Geometry check sheet. Reference: the model listing, model coordinates, mm. A direction names the side the tool comes from. Coordinates: 2 decimals unless noted, no trailing zeros. Order: outer loops, then holes, each group sorted by start corner. A loop starts at its lowest first (then second) coordinate and runs counter-clockwise, first axis right, second up. Notation, with made-up numbers: (8.5, 77) - (56.5, 77) arc R25 cw to (56.5, 102) - close; hole circle Ø7 at (-33.75, 38). An arc over 180 degrees is marked (long way). Return JSON: item names as keys, results as strings. Group by question number.
Item 1: Section check D-D on x = -18. Enter the section's corners in (y, z) (3 decimals), then the cut area to 3 significant figures.
Item 2: Gauge pin test, flat ends, axial feed: pin 1 (2.5 mm diameter, centred on y = 15.5, z = -6.5, fed in from +X); pin 2 (1.7 mm diameter, centred on x = 2.5, y = 4, fed in from +Z); pin 3 (8 mm diameter, centred on y = 20.5, z = 6, fed in from -X); pin 4 (12 mm diameter, centred on x = 6.5, z = -6.5, fed in from -Y). Record the tip position at first contact, or that the pin passes through.
Item 3: Section check B-B on y = 6.75. Enter the section's corners in (x, z) (3 decimals).
Item 4: Draft check along X on faces 6 (the cylindrical face through (-21.555, 5.114, -19.879)), 7 (the flat face through (23, 1, -20.5)), 8 (the cylindrical face through (26.886, 1.166, -0.208)), 9 (the flat face through (28.3, 1, 0)). Enter one of: pulls with the +X half, pulls with the -X half, needs draft (parallel to the pull), parting line crosses it, or undercut.
Item 5: Scan lines: probe 1 along Y at (x, z) = (-24.5, -6.5); probe 2 along X at (y, z) = (1.4, -17.5); probe 3 along Z at (x, y) = (-15, 6). Record each from-to range of solid material in increasing order.
Item 6: Section check C-C on z = -17.5. Enter the section's corners in (x, y) (3 decimals), then the cut area to 3 significant figures.
Item 7: Tool access check on faces 1 (the cylindrical face through (23.237, 5.114, 3.452)), 2 (the flat face through (-21.693, 12.255, 3.512)), 3 (the flat face through (23, 1, 20.5)), 4 (the flat face through (-25, 5, -13.02)), 5 (the flat face through (-22.125, 5, 17)). Record the directions out of +Z, -Z, +X, -X, +Y, -Y that give a thin tool (end or side, any length) a straight path to the whole face; none if there is none.
Item 8: Section check A-A on x = -25.3. Enter the section's corners in (y, z) (3 decimals).
from build123d import *

# Parameters (mm, degrees)
SKETCH1_W               = 56.6
SKETCH1_H               = 41
BOSS_EXTRUDE1_DEPTH     = 2.3
BOSS_EXTRUDE2_DEPTH     = 5.55
BOSS_EXTRUDE3_DEPTH     = 15.15
FILLET1_R               = 2
BOSS_EXTRUDE5_DEPTH     = 2.3
BOSS_EXTRUDE6_DEPTH     = 2.3
SKETCH6_R               = 1.6
CUT_EXTRUDE1_DEPTH      = 42.199956917
FILLET2_R               = 3.5
SKETCH7_R               = 4.708157521
BOSS_EXTRUDE7_DEPTH     = 0.2
SKETCH11_R              = 4.425
BOSS_EXTRUDE8_DEPTH     = 2.45
CUT_EXTRUDE2_DEPTH      = 10
CUT_EXTRUDE2_DEPTH_BACK = 2.45
SKETCH12_R              = 3.925
BOSS_EXTRUDE10_DEPTH    = 1


with BuildPart() as part:
    # Sketch1 → Boss-Extrude1 (new body)
    with BuildSketch(Plane(origin=(0, 0, 0), x_dir=(1, 0, 0), z_dir=(0, 1, 0))):
        Rectangle(SKETCH1_W, SKETCH1_H)
    extrude(amount=BOSS_EXTRUDE1_DEPTH)

    # Sketch2 → Boss-Extrude2 (add)
    with BuildSketch(Plane(origin=(0, 2.3, 0), x_dir=(1, 0, 0), z_dir=(0, 1, 0))):
        Polygon((-22.125, -20.48), (28.285, -20.48), (28.285, -4.45), (22.185, -4.45), (22.185, 4.45), (28.285, 4.45), (28.285, 20.48), (-22.125, 20.48), (-22.125, 13.02), (-28.285, 13.02), (-28.285, -13.02), (-22.125, -13.02), align=None)
    extrude(amount=BOSS_EXTRUDE2_DEPTH)

    # Sketch3 → Boss-Extrude3 (add)
    with BuildSketch(Plane(origin=(0, 7.85, 0), x_dir=(1, 0, 0), z_dir=(0, 1, 0))):
        with BuildLine():
            Line((-19, -18.225), (21, -18.225))
            ThreePointArc((21, -18.225), (22.185, 0), (21, 18.225))
            Line((21, 18.225), (-19, 18.225))
            ThreePointArc((-19, 18.225), (-20.414213562, 17.639213562), (-21, 16.225))
            Line((-21, 16.225), (-21, -16.225))
            ThreePointArc((-21, -16.225), (-20.414213562, -17.639213562), (-19, -18.225))
        make_face()
    extrude(amount=BOSS_EXTRUDE3_DEPTH)

    # Fillet1
    fillet1_edges = [part.edges().sort_by_distance(p)[0] for p in [
        (28.285, 5.075, -20.48),
        (-22.125, 5.075, -20.48),
        (-22.125, 5.075, -13.02),
        (-28.285, 5.075, -13.02),
        (-28.285, 5.075, 13.02),
        (-22.125, 5.075, 13.02),
        (-22.125, 5.075, 20.48),
        (28.285, 5.075, 20.48),
        (28.3, 1.15, 20.5),
        (-28.3, 1.15, 20.5),
        (-28.3, 1.15, -20.5),
        (28.3, 1.15, -20.5),
    ]]
    fillet(fillet1_edges, radius=FILLET1_R)

    # Sketch4 → Boss-Extrude5 (add)
    with BuildSketch(Plane(origin=(0, 0, 0), x_dir=(1, 0, 0), z_dir=(0, 1, 0))):
        with BuildLine():
            Line((28.3, 14.772353725), (28.3, 9.587646275))
            ThreePointArc((28.3, 9.587646275), (28.429084519, 10.095465182), (28.785, 10.48))
            Line((28.785, 10.48), (28.785, 13.88))
            ThreePointArc((28.785, 13.88), (28.429084519, 14.264534818), (28.3, 14.772353725))
        make_face()
        with BuildLine():
            ThreePointArc((28.3, -9.587646275), (28.429084519, -10.095465182), (28.785, -10.48))
            Line((28.785, -10.48), (28.785, -13.88))
            ThreePointArc((28.785, -13.88), (28.429084519, -14.264534818), (28.3, -14.772353725))
            Line((28.3, -14.772353725), (28.3, -9.587646275))
        make_face()
    extrude(amount=BOSS_EXTRUDE5_DEPTH)

    # Sketch5 → Boss-Extrude6 (add)
    with BuildSketch(Plane(origin=(29.434734965, 0, -17.005006325), x_dir=(0, 0, -1), z_dir=(0, 1, 0))):
        with BuildLine():
            Line((3.494993675, 9.629302498), (3.494993675, 9.486266265))
            ThreePointArc((3.494993675, 9.486266265), (3.620682756, 10.143155137), (3.979993675, 10.707244136))
            Line((3.979993675, 10.707244136), (3.979993675, 14.149734965))
            ThreePointArc((3.979993675, 14.149734965), (3.621827878, 14.636664087), (3.494993675, 15.227676603))
            Line((3.494993675, 15.227676603), (3.494993675, 9.629302498))
        make_face()
        with BuildLine():
            Line((-37.505006325, 46.813203664), (-37.505006325, 46.670167432))
            Line((-37.505006325, 46.670167432), (-37.505006325, 41.071793326))
            ThreePointArc((-37.505006325, 41.071793326), (-37.631840527, 41.662805842), (-37.990006325, 42.149734965))
            Line((-37.990006325, 42.149734965), (-37.990006325, 45.592225793))
            ThreePointArc((-37.990006325, 45.592225793), (-37.630695406, 46.156314792), (-37.505006325, 46.813203664))
        make_face()
        with BuildLine():
            Line((3.494993675, 41.071793326), (3.494993675, 46.670167432))
            Line((3.494993675, 46.670167432), (3.494993675, 46.813203664))
            ThreePointArc((3.494993675, 46.813203664), (3.620682756, 46.156314792), (3.979993675, 45.592225793))
            Line((3.979993675, 45.592225793), (3.979993675, 42.149734965))
            ThreePointArc((3.979993675, 42.149734965), (3.621827878, 41.662805842), (3.494993675, 41.071793326))
        make_face()
        with BuildLine():
            Line((-37.505006325, 15.227676603), (-37.505006325, 9.629302498))
            Line((-37.505006325, 9.629302498), (-37.505006325, 9.486266265))
            ThreePointArc((-37.505006325, 9.486266265), (-37.630695406, 10.143155137), (-37.990006325, 10.707244136))
            Line((-37.990006325, 10.707244136), (-37.990006325, 14.149734965))
            ThreePointArc((-37.990006325, 14.149734965), (-37.631840527, 14.636664087), (-37.505006325, 15.227676603))
        make_face()
    extrude(amount=BOSS_EXTRUDE6_DEPTH)

    # Sketch6 → Cut-Extrude1 (cut, through all)
    with BuildSketch(Plane(origin=(0, 2.3, 0), x_dir=(1, 0, 0), z_dir=(0, 1, 0))):
        with Locations(Location((-25.3, 17.5, 0), (0, 0, 270))):
            Circle(SKETCH6_R)
        with Locations(Location((-25.3, -17.5, 0), (0, 0, 90))):
            Circle(SKETCH6_R)
        with Locations(Location((25.3, 0, 0), (0, 0, 270))):
            Circle(SKETCH6_R)
    extrude(amount=-CUT_EXTRUDE1_DEPTH, mode=Mode.SUBTRACT)

    # Fillet2
    fillet2_edges = [part.edges().sort_by_distance(p)[0] for p in [
        (22.185, 5.075, 4.45),
        (22.185, 5.075, -4.45),
    ]]
    fillet(fillet2_edges, radius=FILLET2_R)

    # Sketch7 → Boss-Extrude7 (add)
    with BuildSketch(Plane.ZY.offset(21)):
        with Locations(Location((7.06, 14.265, 0), (0, 0, 180))):
            Circle(SKETCH7_R)
    extrude(amount=BOSS_EXTRUDE7_DEPTH)

    # Sketch9 → Revolve1 (revolve)
    with BuildSketch(Plane(origin=(0, 0, -6.66), x_dir=(-1, 0, 0), z_dir=(0, 0, -1))):
        Polygon((21, 20.396842479), (21, 14.265), (24, 14.265), (24, 18.665), (22.15, 20.396842479), align=None)
    revolve(axis=Axis((-21, 14.265, -6.66), (-1, 0, 0)))

    # Sketch11 → Boss-Extrude8 (add)
    with BuildSketch(Plane.ZY.offset(24)):
        with Locations(Location((-6.66, 14.265, 0), (0, 0, 270))):
            Circle(SKETCH11_R)
    extrude(amount=BOSS_EXTRUDE8_DEPTH)

    # Sketch12 → Cut-Extrude2 (cut, two sides: drawn at the far end of the back side and taken through both)
    with BuildSketch(Plane.ZY.offset(26.45).offset(-CUT_EXTRUDE2_DEPTH_BACK)):
        with Locations(Location((-6.66, 14.265, 0), (0, 0, 270))):
            Circle(SKETCH12_R)
    extrude(amount=CUT_EXTRUDE2_DEPTH + CUT_EXTRUDE2_DEPTH_BACK, mode=Mode.SUBTRACT)

    # Sketch13 → Boss-Extrude10 (add)
    with BuildSketch(Plane.ZY.offset(21.2)):
        Polygon((2.351842479, 14.265), (4.705921239, 10.187615982), (9.414078761, 10.187615982), (11.768157521, 14.265), (9.414078761, 18.342384018), (4.705921239, 18.342384018), align=None)
    extrude(amount=BOSS_EXTRUDE10_DEPTH)


solid = part.part
Computed:
{
 "1": {"outline": "(0, -20.5) - (2.3, -20.5) - (2.3, -20.48) - (7.85, -20.48) - (7.85, -18.225) - (23, -18.225) - (23, 18.225) - (7.85, 18.225) - (7.85, 20.48) - (2.3, 20.48) - (2.3, 20.5) - (0, 20.5) - close", "area": "874 mm²"},
 "2": {"pin 1": "stops at x = 22.09", "pin 2": "stops at z = 20.48", "pin 3": "stops at x = -22.2", "pin 4": "stops at y = 0"},
 "3": {"outline": "(-28.285, -11.02) arc R2 ccw to (-26.285, -13.02) - (-24.125, -13.02) arc R2 cw to (-22.125, -15.02) - (-22.125, -18.48) arc R2 ccw to (-20.125, -20.48) - (26.285, -20.48) arc R2 ccw to (28.285, -18.48) - (28.285, -4.45) - (25.685, -4.45) arc R3.5 cw to (22.185, -0.95) - (22.185, 0.95) arc R3.5 cw to (25.685, 4.45) - (28.285, 4.45) - (28.285, 18.48) arc R2 ccw to (26.285, 20.48) - (-20.125, 20.48) arc R2 ccw to (-22.125, 18.48) - (-22.125, 15.02) arc R2 cw to (-24.125, 13.02) - (-26.285, 13.02) arc R2 ccw to (-28.285, 11.02) - close"},
 "4": {"face 6": "pulls with the -X half", "face 7": "needs draft", "face 8": "undercut", "face 9": "pulls with the +X half"},
 "5": {"probe 1": "y = 0 to 7.85, 9.84 to 10.34, 18.19 to 18.69", "probe 2": "x = -28.3 to -26.9, -23.7 to 28.3", "probe 3": "z = -20.48 to 20.48"},
 "6": {"outline": "(-28.3, 0) - (-26.9, 0) - (-26.9, 2.3) - (-28.3, 2.3) - close; (-23.7, 0) - (28.3, 0) - (28.3, 2.3) - (28.285, 2.3) - (28.285, 7.85) - (21.093, 7.85) - (21.093, 23) - (-20.541, 23) - (-20.541, 7.85) - (-22.125, 7.85) - (-22.125, 2.3) - (-23.7, 2.3) - close", "area": "1,030 mm²"},
 "7": {"face 1": "+X, +Y", "face 2": "-X", "face 3": "+Z, +X, +Y, -Y", "face 4": "-Z, -X, +Y", "face 5": "+Z, -X, +Y"},
 "8": {"outline": "(0, -20.5) - (2.3, -20.5) - (2.3, -19.1) - (0, -19.1) - close; (0, -15.9) - (2.3, -15.9) - (2.3, -13.02) - (7.85, -13.02) - (7.85, 13.02) - (2.3, 13.02) - (2.3, 15.9) - (0, 15.9) - close; (0, 19.1) - (2.3, 19.1) - (2.3, 20.5) - (0, 20.5) - close; circle Ø8.85 at (14.265, -6.66); hole circle Ø7.85 at (14.265, -6.66)"}
}
